Could you check a few things on this model? Use its own coordinates, in mm. A direction names the side the tool comes from. Round coordinates to 2 decimals unless told otherwise and drop trailing zeros. Order: outer loops, then holes, each group sorted by start corner. A loop starts at its lowest first (then second) coordinate and runs counter-clockwise, first axis right, second up. Notation, with made-up numbers: (5.5, -18) -> (35.5, -18) arc R18 cw to (35.5, 10) -> close; hole circle Ø9 at (-39.5, 17.5). An arc over 180 degrees is marked (long way). Put each result on its own line as item: value. Start each with the question number.
from build123d import *

# Parameters (mm, degrees)
SKETCH1_W           = 6
SKETCH1_H           = 10
SKETCH1_R           = 1.5
BOSS_EXTRUDE1_DEPTH = 10
SKETCH2_W           = 3.2
SKETCH2_H           = 3.2
CUT_EXTRUDE1_DEPTH  = 16.362291496
SKETCH1_3_R         = 1.5
BOSS_EXTRUDE2_DEPTH = 3.4


with BuildPart() as part:
    # Sketch1 → Boss-Extrude1 (new body)
    with BuildSketch(Plane.XY):
        with Locations((3, 5)):
            Rectangle(SKETCH1_W, SKETCH1_H)
        with Locations((3, 5)):
            Circle(SKETCH1_R, mode=Mode.SUBTRACT)
    extrude(amount=BOSS_EXTRUDE1_DEPTH)

    # Sketch2 → Cut-Extrude1 (cut, through all)
    with BuildSketch(Plane(origin=(6, 0, 0), x_dir=(0, 0, -1), z_dir=(1, 0, 0))):
        with Locations((-5, 5)):
            Rectangle(SKETCH2_W, SKETCH2_H)
    extrude(amount=-CUT_EXTRUDE1_DEPTH, mode=Mode.SUBTRACT)

    # Sketch1<3> → Boss-Extrude2 (add)
    with BuildSketch(Plane.XY):
        with Locations((3, 5)):
            Circle(SKETCH1_3_R)
        Polygon((0, 10), (6, 0), (0, 0), align=None)
        Polygon((0, 10), (6, 10), (6, 0), align=None)
    extrude(amount=BOSS_EXTRUDE2_DEPTH)


solid = part.part
1. If we section it at D-D, the plane x = 3: Please give me the cut outline in (y, z).
2. If we section it at B-B, the plane x = 5.05: Please give me the cut outline in (y, z), then the cut area to 3 significant figures.
3. For pin 1 Ø2.5 at (x, y) = (3, 5) entering from +Z, with a flat end and sliding along its axis, tell me the tip position at first contact or that it passes through.
4. I need wall thicknesses on L1, parallel to Y at x = 4.75, z = 5.75; L2, parallel to X at y = 5, z = 8; L3, parallel to Y at x = 3, z = 7.75. Which ranges of each line are inside material? Lowest first, please.
5. If we section it at C-C, the plane z = 4.5: Please give me the cut outline in (x, y).
6. Which directions (+Z, -Z, +X, -X, +Y, -Y) give clear straight access to the entire face, cutting with the end or side of a thin tool? Please do faces 4 (the face through (3, 6.6, 5)), 5 (the face through (6, 7, 5)), 6 (the face through (4.386, 4.425, 8.276)).
7. Thinking about a two-plate mould opening in Y: for faces 1 (the face through (0, 7, 5)), 2 (the face through (3, 5, 3.4)), 3 (the face through (3, 0, 5)), which applies, +Y half, -Y half, draft (parallel to the pull), parting line (faces both ways), or undercut?
8. If we section it at A-A, the plane y = 5: Please give me the cut outline in (x, z), then the cut area to 3 significant figures.
Results below:
1. outline: (0, 0) -> (10, 0) -> (10, 10) -> (6.5, 10) -> (6.5, 6.6) -> (6.6, 6.6) -> (6.6, 3.4) -> (3.4, 3.4) -> (3.4, 6.6) -> (3.5, 6.6) -> (3.5, 10) -> (0, 10) -> close
2. outline: (0, 0) -> (10, 0) -> (10, 10) -> (0, 10) -> close; hole (3.4, 3.4) -> (6.6, 3.4) -> (6.6, 6.6) -> (3.4, 6.6) -> close
2. area: 89.8 mm2
3. pin 1: z = 3.4
4. L1: 0 to 3.4, 6.6 to 10
4. L2: 0 to 1.5, 4.5 to 6
4. L3: 0 to 3.5, 6.5 to 10
5. outline: (0, 0) -> (6, 0) -> (6, 3.4) -> (0, 3.4) -> close; (0, 6.6) -> (6, 6.6) -> (6, 10) -> (0, 10) -> close
6. face 4: +X, -X
6. face 5: +Z, -Z, +X, +Y, -Y
6. face 6: +Z
7. face 1: draft
7. face 2: undercut
7. face 3: -Y half
8. outline: (0, 0) -> (6, 0) -> (6, 3.4) -> (0, 3.4) -> close; (0, 6.6) -> (1.5, 6.6) -> (1.5, 10) -> (0, 10) -> close; (4.5, 6.6) -> (6, 6.6) -> (6, 10) -> (4.5, 10) -> close
8. area: 30.6 mm2
